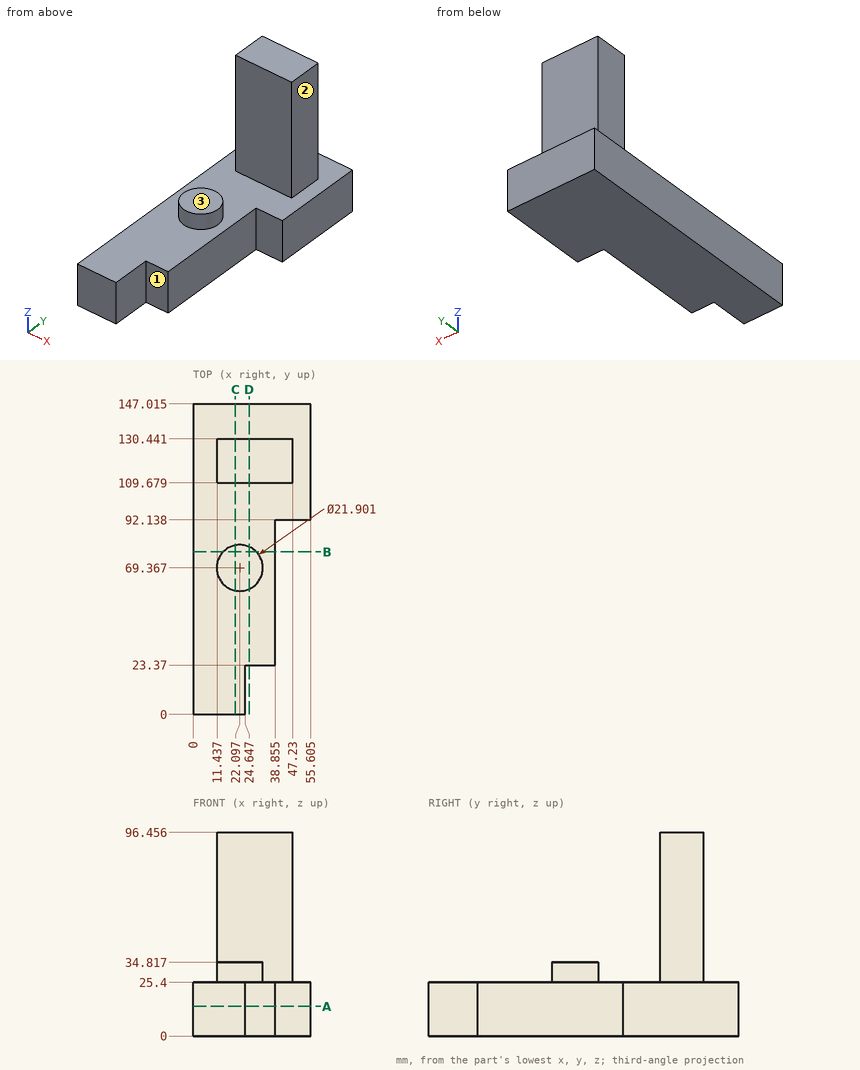
Design review of the part shown in the three views and the two pictorial views. Dimensions are in mm from the part's minimum x, y and z. A direction names the side the tool comes from. Coordinates: 2 decimals unless noted, no trailing zeros. Order: outer loops, then holes, each group sorted by start corner. A loop starts at its lowest first (then second) coordinate and runs counter-clockwise, first axis right, second up.
Item 1: Take a section at A-A, the plane z = 14. Write out the cut boundary in (x, y) (1 decimal), then the cut area to 3 significant figures.
Item 2: Take a section at B-B, the plane y = 77. Write out the cut boundary in (x, z) (1 decimal).
Item 3: For the marked faces 1, 2 and 3, list the 3-axis set-ups (+Z, -Z, +X, -X, +Y, -Y) from which the entire face can be reached by the end or side of a thin tool; tool diameter is ignored.
Item 4: Take a section at C-C, the plane x = 20. Write out the cut boundary in (y, z) (1 decimal).
Item 5: For pin 1 Ø18 at (x, z) = (37, 64) entering from +Y; pin 2 Ø10.5 at (x, z) = (26, 72.5) entering from -Y; pin 3 Ø23 at (y, z) = (117, 78) entering from -X; pin 4 Ø4 at (x, y) = (41.5, 30.5) entering from -Z, all flat-tipped, find the tip position at first contact; note any pin that passes through.
Item 6: Take a section at D-D, the plane x = 26.5. Write out the cut boundary in (y, z) (1 decimal).
Item 7: For line 1 (Y direction, x = 45.5, z = 48.5); line 2 (X direction, y = 114.5, z = 43.5); line 3 (Y direction, x = 48, z = 24) (1 decimal), list the stretches that pass through material, from the lowest coordinate up.
The answers:
1. outline: (0, 0) - (24.6, 0) - (24.6, 23.4) - (38.9, 23.4) - (38.9, 92.1) - (55.6, 92.1) - (55.6, 147) - (0, 147) - close
1. area: 6,300 mm2
2. outline: (0, 0) - (38.9, 0) - (38.9, 25.4) - (29.9, 25.4) - (29.9, 34.8) - (14.2, 34.8) - (14.2, 25.4) - (0, 25.4) - close
3. face 1: +Z, -Z, +X, -Y
3. face 2: +Z, +X, +Y, -Y
3. face 3: +Z, +X, -X, -Y
4. outline: (0, 0) - (147, 0) - (147, 25.4) - (130.4, 25.4) - (130.4, 96.5) - (109.7, 96.5) - (109.7, 25.4) - (80.1, 25.4) - (80.1, 34.8) - (58.6, 34.8) - (58.6, 25.4) - (0, 25.4) - close
5. pin 1: stops at y = 130.44
5. pin 2: stops at y = 109.68
5. pin 3: stops at x = 11.44
5. pin 4: passes through
6. outline: (23.4, 0) - (147, 0) - (147, 25.4) - (130.4, 25.4) - (130.4, 96.5) - (109.7, 96.5) - (109.7, 25.4) - (79.4, 25.4) - (79.4, 34.8) - (59.3, 34.8) - (59.3, 25.4) - (23.4, 25.4) - close
7. line 1: y = 109.68 to 130.44
7. line 2: x = 11.44 to 47.23
7. line 3: y = 92.1 to 147
